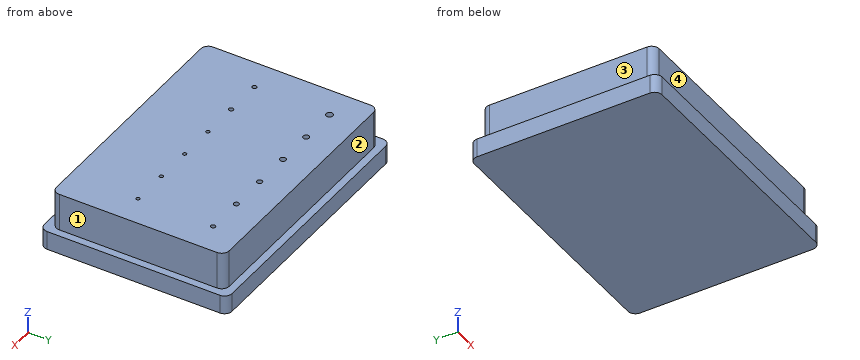
```python
from build123d import *

# Parameters (mm, degrees)
F0_W     = 70
F0_H     = 50
F1_DEPTH = 5
F2_W     = 66
F2_H     = 46
F3_DEPTH = 10
F4_R     = 2
F5_R     = 0.5
F5_R_2   = 0.6
F5_R_3   = 0.7
F5_R_4   = 0.8
F5_R_5   = 0.9
F6_DEPTH = 10


with BuildPart() as f1:
    # F0 (on Top) → F1 (new body)
    with BuildSketch(Plane.XY):
        Rectangle(F0_W, F0_H)
    extrude(amount=F1_DEPTH)

    # F2 (on face) → F3 (join)
    with BuildSketch(Plane.XY.offset(5)):
        Rectangle(F2_W, F2_H)
    extrude(amount=F3_DEPTH)

    # F4
    f4_edges = [f1.edges().sort_by_distance(p)[0] for p in [
        (-33, -23, 10),
        (33, -23, 10),
        (35, -25, 2.5),
        (-35, -25, 2.5),
        (-35, 25, 2.5),
        (-33, 23, 10),
        (33, 23, 10),
        (35, 25, 2.5),
    ]]
    fillet(f4_edges, radius=F4_R)

    # F5 (on face) → F6 (cut)
    with BuildSketch(Plane.XY.offset(15)):
        with Locations((25, -5)):
            Circle(F5_R)
        with Locations((15, -5)):
            Circle(F5_R)
        with Locations((5, -5)):
            Circle(F5_R)
        with Locations((-5, -5)):
            Circle(F5_R)
        with Locations((-15, -5)):
            Circle(F5_R_2)
        with Locations((-25, -5)):
            Circle(F5_R_2)
        with Locations((25, 15)):
            Circle(F5_R_2)
        with Locations((15, 15)):
            Circle(F5_R_3)
        with Locations((5, 15)):
            Circle(F5_R_3)
        with Locations((-5, 15)):
            Circle(F5_R_4)
        with Locations((-15, 15)):
            Circle(F5_R_4)
        with Locations((-25, 15)):
            Circle(F5_R_5)
    extrude(amount=-F6_DEPTH, mode=Mode.SUBTRACT)


solid = f1.part
```
The model under review builds one solid part; all positions refer to its coordinate system, in mm. Face numbers are marked on the shaded views. A direction names the side the tool comes from. Give positions to 0.01 mm unless a question says otherwise; leave off trailing zeros. Write each loop counter-clockwise with the first axis right and the second up, starting at its lowest first coordinate (ties: lowest second). Pieces come first, ordered by that corner, then holes. Notation, with made-up numbers: M -34,80 L -3,80 A11 cw -3,93 Z; hole C 24,35 d2. An arc over 180 degrees is marked long. Write each question's results on one line, items separated by ' | '. Start each with the question number.
1. For the marked faces 1, 2, 3 and 4, list the 3-axis set-ups (+Z, -Z, +X, -X, +Y, -Y) from which the entire face can be reached by the end or side of a thin tool; tool diameter is ignored.
2. Insertion check: pin 1 Ø0.8 at (x, y) = (-5, -5) entering from +Z; pin 2 Ø1.5 at (y, z) = (6.5, 9) entering from +X; pin 3 Ø5 at (x, z) = (-4, 10) entering from -Y. Each pin has a flat end and moves straight along its axis. Give the tip position at first contact, or say it passes through.
3. For probe 1 along Y at (x, z) = (25, 11); probe 2 along Y at (x, z) = (-5, 12.25); probe 3 along X at (y, z) = (2, 6.25), list the stretches that pass through material, from the lowest coordinate up. Write a range as [from, to].
4. We need section A-A (z = 13.5). Count the separate pieces of the cut face and the enclosed holes in it, and give its area (3 significant figures).
5. We need section B-B (y = 11). Write out the cut boundary in (x, z).
6. We need section C-C (x = -21.5). Write out the cut boundary in (y, z).
Results found:
1) face 1: +Z, +X, +Y, -Y | face 2: +Z, +X, -X, +Y | face 3: +Z, -X, +Y, -Y | face 4: +Z, +X, -X, -Y
2) pin 1: stops at z = 5 | pin 2: stops at x = 33 | pin 3: stops at y = -23
3) probe 1: y = [-23, -5.5], [-4.5, 14.4], [15.6, 23] | probe 2: y = [-23, -5.5], [-4.5, 14.2], [15.8, 23] | probe 3: x = [-33, 33]
4) separate pieces: 1 | enclosed holes: 12 | area: 3,020 mm^2
5) outline: M -35,0 L 35,0 L 35,5 L 33,5 L 33,15 L -33,15 L -33,5 L -35,5 Z
6) outline: M -25,0 L 25,0 L 25,5 L 23,5 L 23,15 L -23,15 L -23,5 L -25,5 Z
